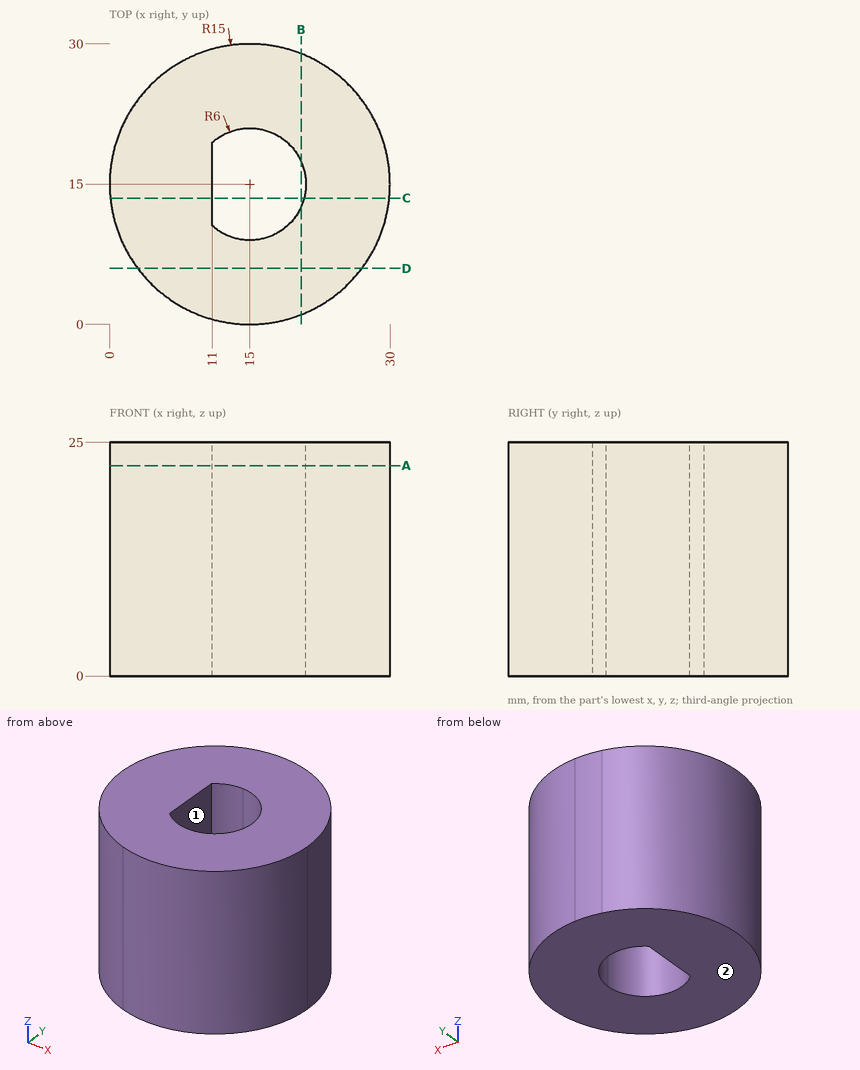
Can you work these out from the drawing? Everything is in mm from the part's minimum corner. Give positions to 0.01 mm unless a question says otherwise; leave off trailing zeros. Order: outer loops, then holes, each group sorted by start corner. A loop starts at its lowest first (then second) coordinate and runs counter-clockwise, first axis right, second up.
Item 1: If we section it at C-C, the plane y = 13.5: Write out the boundary of the cut face in (x, z).
Item 2: I need wall thicknesses on line 1 (Y direction, x = 19, z = 6); line 2 (X direction, y = 11, z = 8.5); line 3 (X direction, y = 15, z = 6.5). Which ranges of each line are inside material? Lowest first, please.
Item 3: If we section it at A-A, the plane z = 22.5: Write out the boundary of the cut face in (x, y), plus the area to 3 significant figures.
Item 4: If we section it at B-B, the plane x = 20.5: Write out the boundary of the cut face in (y, z), plus the area to 3 significant figures.
Item 5: I'm going to push flat-ended pins straight in: pin 1 (1.5 mm diameter, centred on y = 11.5, z = 11.5, fed in from +X); pin 2 (8 mm diameter, centred on x = 8.5, z = 18, fed in from +Y); pin 3 (1 mm diameter, centred on x = 21, z = 16, fed in from -Y). Where does each tip first touch, or does it pass through?
Item 6: If we section it at D-D, the plane y = 6: Write out the boundary of the cut face in (x, z), plus the area to 3 significant figures.
Item 7: If we mould it in two halves opening along X, with no side actions, what happens to the marked faces 1 and 2? For each: pulls with the +X half, pulls with the -X half, needs draft (parallel to the pull), parting line crosses it, or undercut.
Values:
1. outline: (0.08, 0) - (11, 0) - (11, 25) - (0.08, 25) - close; (20.81, 0) - (29.92, 0) - (29.92, 25) - (20.81, 25) - close
2. line 1: y = 0.54 to 10.53, 19.47 to 29.46
2. line 2: x = 0.54 to 11, 19.47 to 29.46
2. line 3: x = 0 to 11, 21 to 30
3. outline: circle Ø30 at (15, 15); hole (11, 10.53) arc R6 ccw (long way) to (11, 19.47) - close
3. area: 606 mm2
4. outline: (1.04, 0) - (12.6, 0) - (12.6, 25) - (1.04, 25) - close; (17.4, 0) - (28.96, 0) - (28.96, 25) - (17.4, 25) - close
4. area: 578 mm2
5. pin 1: stops at x = 29.75
5. pin 2: stops at y = 29.79
5. pin 3: stops at y = 1.04
6. outline: (3, 0) - (27, 0) - (27, 25) - (3, 25) - close
6. area: 600 mm2
7. face 1: undercut
7. face 2: needs draft
